from build123d import *

# Parameters (mm, degrees)
F0_W     = 300
F0_H     = 400
F1_DEPTH = 19
F2_W     = 278
F2_H     = 46
F3_DEPTH = 10
F4_W     = 30
F4_H     = 46
F5_DEPTH = 10
F6_W     = 260
F6_H     = 312
F7_DEPTH = 10


with BuildPart() as f1:
    # F0 (on Front) → F1 (new body)
    with BuildSketch(Plane.XZ):
        with Locations((-8.346558, 189.359199)):
            Rectangle(F0_W, F0_H)
    extrude(amount=F1_DEPTH)

    # F2 (on face) → F3 (cut)
    with BuildSketch(Plane(origin=(0, 0, 0), x_dir=(-1, 0, 0), z_dir=(0, 1, 0))):
        with Locations((8.846558, 356.359199)):
            Rectangle(F2_W, F2_H)
    extrude(amount=-F3_DEPTH, mode=Mode.SUBTRACT)

    # F4 (on face) → F5 (cut)
    with BuildSketch(Plane(origin=(0, -10, 0), x_dir=(-1, 0, 0), z_dir=(0, 1, 0))):
        with Locations((132.846558, 356.359199)):
            Rectangle(F4_W, F4_H)
    extrude(amount=-F5_DEPTH, mode=Mode.SUBTRACT)

    # F6 (on face) → F7 (cut)
    with BuildSketch(Plane(origin=(0, 0, 0), x_dir=(-1, 0, 0), z_dir=(0, 1, 0))):
        with Locations((8.346558, 167.359199)):
            Rectangle(F6_W, F6_H)
    extrude(amount=-F7_DEPTH, mode=Mode.SUBTRACT)


solid = f1.part
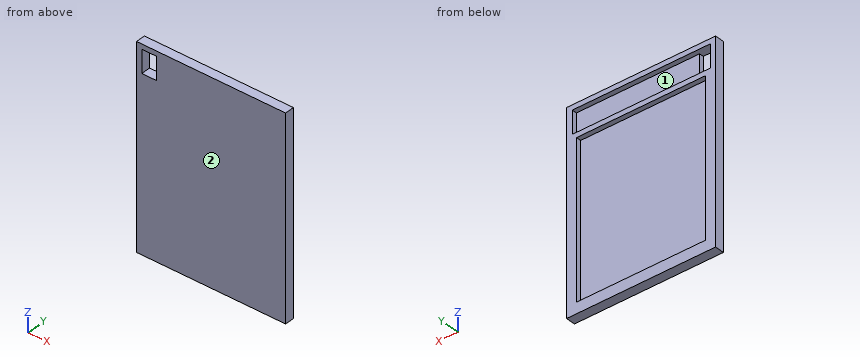
Input: part model. Units: mm. Frame: model coordinates. Face numbers are marked on the shaded views. Give positions to 0.01 mm unless a question says otherwise; leave off trailing zeros. Write each loop counter-clockwise with the first axis right and the second up, starting at its lowest first coordinate (ties: lowest second). Pieces come first, ordered by that corner, then holes. Notation, with made-up numbers: (62, 82) -> (70, 82) arc R27 cw to (70, 105) -> close; hole circle Ø7 at (41, -1). An arc over 180 degrees is marked (long way). Use one line per item in the form item = value. Start each with the question number.
1) Ray query, probe 1 along Z at (x, y) = (3, -3); probe 2 along X at (y, z) = (-6.25, 310); probe 3 along X at (y, z) = (-17.75, 367.5). Return the intervals inside material, ascending. Write a range as from..to.
2) Draft query along X for the marked faces 1 and 2. Return one class per face: pulls with the +X half, pulls with the -X half, needs draft (parallel to the pull), parting line crosses it, or undercut.
3) Section query A-A on y = -6. Return the cut outline in (x, z).
4) Pin query (flat end, axial travel): pin 1 (10 mm diameter, centred on x = 87, z = 97.5, fed in from +Y). Return the tip coordinate at first contact, or that it passes through.
5) Section query B-B on z = 289.5. Return the cut outline in (x, y), then the cut area to 3 significant figures.
6) Section query C-C on x = 4. Return the cut outline in (y, z).
Outcome:
q1.probe_1 = -10.64..11.36, 323.36..333.36, 379.36..389.36
q1.probe_2 = -158.35..-138.35, 121.65..141.65
q1.probe_3 = -158.35..-147.85, -117.85..141.65
q2.face_1 = undercut
q2.face_2 = needs draft
q3.outline = (-158.35, -10.64) -> (141.65, -10.64) -> (141.65, 389.36) -> (-158.35, 389.36) -> close; hole (-147.85, 333.36) -> (130.15, 333.36) -> (130.15, 379.36) -> (-147.85, 379.36) -> close; hole (-138.35, 11.36) -> (121.65, 11.36) -> (121.65, 323.36) -> (-138.35, 323.36) -> close
q4.pin_1 = -10
q5.outline = (-158.35, -19) -> (141.65, -19) -> (141.65, 0) -> (121.65, 0) -> (121.65, -10) -> (-138.35, -10) -> (-138.35, 0) -> (-158.35, 0) -> close
q5.area = 3,100 mm^2
q6.outline = (-19, -10.64) -> (0, -10.64) -> (0, 11.36) -> (-10, 11.36) -> (-10, 323.36) -> (0, 323.36) -> (0, 333.36) -> (-10, 333.36) -> (-10, 379.36) -> (0, 379.36) -> (0, 389.36) -> (-19, 389.36) -> close
